Build history of the part. All positions in model axes, mm. A direction names the side the tool comes from. Give positions to 0.01 mm unless a question says otherwise; leave off trailing zeros. Order: outer loops, then holes, each group sorted by start corner. A loop starts at its lowest first (then second) coordinate and runs counter-clockwise, first axis right, second up. Notation, with made-up numbers: M -14.75,-11 L 26.25,-11 A9 ccw 26.25,-6 Z; hole C -38,40.5 d1. An arc over 180 degrees is marked long. Answer as CSV lines item,"result".
from build123d import *

# Parameters (mm, degrees)
RESSALTO_EXTRUS_O3_DEPTH = 5
ESBO_O4_R                = 1.5
CORTE_EXTRUS_O3_DEPTH    = 10
CORTE_EXTRUS_O4_DEPTH    = 10


with BuildPart() as part:
    # Esboço1 → Ressalto-extrusão3 (new body)
    with BuildSketch(Plane.XY):
        with BuildLine():
            Line((-31.851570772, -17.801096987), (-27.063885949, -17.801096987))
            Line((-27.063885949, -17.801096987), (10.936114051, -17.801096987))
            Line((10.936114051, -17.801096987), (15.723798874, -17.801096987))
            ThreePointArc((15.723798874, -17.801096987), (21.039894205, -19.331201448), (24.729153299, -23.4532709))
            ThreePointArc((24.729153299, -23.4532709), (27.934250919, -27.635644423), (32.536114051, -30.202306605))
            ThreePointArc((32.536114051, -30.202306605), (35.210937986, -29.759166326), (36.436114051, -27.340489001))
            Line((36.436114051, -27.340489001), (36.436114051, -17.801096987))
            Line((36.436114051, -17.801096987), (36.436114051, 0.198903013))
            add(Edge.make_bspline(
                [(36.436114051, 75.398903013), (24.729153299, 37.798903013), (36.436114051, 0.198903013)],
                knots=[0, 0, 0, 1, 1, 1], degree=2, weights=[1, 3, 1]))
            Line((36.436114051, 75.398903013), (36.436114051, 93.398903013))
            Line((36.436114051, 93.398903013), (36.436114051, 102.938295027))
            ThreePointArc((36.436114051, 102.938295027), (35.210937986, 105.356972352), (32.536114051, 105.800112631))
            ThreePointArc((32.536114051, 105.800112631), (27.934250919, 103.23345045), (24.729153299, 99.051076926))
            ThreePointArc((24.729153299, 99.051076926), (21.039894205, 94.929007474), (15.723798874, 93.398903013))
            Line((15.723798874, 93.398903013), (10.936114051, 93.398903013))
            Line((10.936114051, 93.398903013), (-27.063885949, 93.398903013))
            Line((-27.063885949, 93.398903013), (-31.851570772, 93.398903013))
            ThreePointArc((-31.851570772, 93.398903013), (-37.167666102, 94.929007474), (-40.856925197, 99.051076926))
            ThreePointArc((-40.856925197, 99.051076926), (-44.062022817, 103.23345045), (-48.663885949, 105.800112631))
            ThreePointArc((-48.663885949, 105.800112631), (-51.338709884, 105.356972352), (-52.563885949, 102.938295027))
            Line((-52.563885949, 102.938295027), (-52.563885949, 93.398903013))
            Line((-52.563885949, 93.398903013), (-52.563885949, 75.398903013))
            add(Edge.make_bspline(
                [(-52.563885949, 75.398903013), (-40.856925197, 37.798903013), (-52.563885949, 0.198903013)],
                knots=[0, 0, 0, 1, 1, 1], degree=2, weights=[1, 3, 1]))
            Line((-52.563885949, 0.198903013), (-52.563885949, -17.801096987))
            Line((-52.563885949, -17.801096987), (-52.563885949, -27.340489001))
            ThreePointArc((-52.563885949, -27.340489001), (-51.338709884, -29.759166326), (-48.663885949, -30.202306605))
            ThreePointArc((-48.663885949, -30.202306605), (-44.062022817, -27.635644423), (-40.856925197, -23.4532709))
            ThreePointArc((-40.856925197, -23.4532709), (-37.167666102, -19.331201448), (-31.851570772, -17.801096987))
        make_face()
    extrude(amount=RESSALTO_EXTRUS_O3_DEPTH)

    # Esboço4 → Corte-extrusão3 (cut)
    with BuildSketch(Plane(origin=(0, 0, 0), x_dir=(-1, 0, 0), z_dir=(0, 0, -1))):
        with Locations((-31.436114051, 99.800112631)):
            Circle(ESBO_O4_R)
        with Locations((47.563885949, 99.800112631)):
            Circle(ESBO_O4_R)
        with Locations((47.563885949, -24.202306605)):
            Circle(ESBO_O4_R)
        with Locations((-31.436114051, -24.202306605)):
            Circle(ESBO_O4_R)
        with BuildLine():
            Line((-12.436114051, 90.598903013), (-1.436114051, 90.598903013))
            ThreePointArc((-1.436114051, 90.598903013), (-0.021900489, 90.013116575), (0.563885949, 88.598903013))
            Line((0.563885949, 88.598903013), (0.563885949, 78.698903013))
            ThreePointArc((0.563885949, 78.698903013), (-0.021900489, 77.284689451), (-1.436114051, 76.698903013))
            Line((-1.436114051, 76.698903013), (-12.436114051, 76.698903013))
            ThreePointArc((-12.436114051, 76.698903013), (-13.850327613, 77.284689451), (-14.436114051, 78.698903013))
            Line((-14.436114051, 78.698903013), (-14.436114051, 88.598903013))
            ThreePointArc((-14.436114051, 88.598903013), (-13.850327613, 90.013116575), (-12.436114051, 90.598903013))
        make_face()
        with BuildLine():
            Line((17.563885949, 90.598903013), (28.563885949, 90.598903013))
            ThreePointArc((28.563885949, 90.598903013), (29.978099511, 90.013116575), (30.563885949, 88.598903013))
            Line((30.563885949, 88.598903013), (30.563885949, 78.698903013))
            ThreePointArc((30.563885949, 78.698903013), (29.978099511, 77.284689451), (28.563885949, 76.698903013))
            Line((28.563885949, 76.698903013), (17.563885949, 76.698903013))
            ThreePointArc((17.563885949, 76.698903013), (16.149672387, 77.284689451), (15.563885949, 78.698903013))
            Line((15.563885949, 78.698903013), (15.563885949, 88.598903013))
            ThreePointArc((15.563885949, 88.598903013), (16.149672387, 90.013116575), (17.563885949, 90.598903013))
        make_face()
        with BuildLine():
            Line((30.563885949, -13.001096987), (30.563885949, -3.101096987))
            ThreePointArc((30.563885949, -3.101096987), (29.978099511, -1.686883425), (28.563885949, -1.101096987))
            Line((28.563885949, -1.101096987), (17.563885949, -1.101096987))
            ThreePointArc((17.563885949, -1.101096987), (16.149672387, -1.686883425), (15.563885949, -3.101096987))
            Line((15.563885949, -3.101096987), (15.563885949, -13.001096987))
            ThreePointArc((15.563885949, -13.001096987), (16.149672387, -14.415310549), (17.563885949, -15.001096987))
            Line((17.563885949, -15.001096987), (28.563885949, -15.001096987))
            ThreePointArc((28.563885949, -15.001096987), (29.978099511, -14.415310549), (30.563885949, -13.001096987))
        make_face()
        with BuildLine():
            Line((0.563885949, -13.001096987), (0.563885949, -3.101096987))
            ThreePointArc((0.563885949, -3.101096987), (-0.021900489, -1.686883425), (-1.436114051, -1.101096987))
            Line((-1.436114051, -1.101096987), (-12.436114051, -1.101096987))
            ThreePointArc((-12.436114051, -1.101096987), (-13.850327613, -1.686883425), (-14.436114051, -3.101096987))
            Line((-14.436114051, -3.101096987), (-14.436114051, -13.001096987))
            ThreePointArc((-14.436114051, -13.001096987), (-13.850327613, -14.415310549), (-12.436114051, -15.001096987))
            Line((-12.436114051, -15.001096987), (-1.436114051, -15.001096987))
            ThreePointArc((-1.436114051, -15.001096987), (-0.021900489, -14.415310549), (0.563885949, -13.001096987))
        make_face()
    extrude(amount=-CORTE_EXTRUS_O3_DEPTH, mode=Mode.SUBTRACT)

    # Esboço5 → Corte-extrusão4 (cut)
    with BuildSketch(Plane.XY.offset(5)):
        with BuildLine():
            Line((2.436114051, 17.798903013), (12.436114051, 17.798903013))
            ThreePointArc((12.436114051, 17.798903013), (15.971647957, 19.263369107), (17.436114051, 22.798903013))
            Line((17.436114051, 22.798903013), (17.436114051, 52.798903013))
            ThreePointArc((17.436114051, 52.798903013), (15.971647957, 56.334436919), (12.436114051, 57.798903013))
            Line((12.436114051, 57.798903013), (2.436114051, 57.798903013))
            ThreePointArc((2.436114051, 57.798903013), (-1.099419855, 56.334436919), (-2.563885949, 52.798903013))
            Line((-2.563885949, 52.798903013), (-2.563885949, 22.798903013))
            ThreePointArc((-2.563885949, 22.798903013), (-1.099419855, 19.263369107), (2.436114051, 17.798903013))
        make_face()
    extrude(amount=-CORTE_EXTRUS_O4_DEPTH, mode=Mode.SUBTRACT)


solid = part.part
Item 1: Band-saw the part on B-B (y = -8). Give the cut face in (x, z).
Geometry says:
outline,"M -52.56,0 L -30.56,0 L -30.56,5 L -52.56,5 Z; M -15.56,0 L -0.56,0 L -0.56,5 L -15.56,5 Z; M 14.44,0 L 36.44,0 L 36.44,5 L 14.44,5 Z"
Item 2: 3-axis set-ups, long thin cutter, end or side, ignore diameter. For faces 4 (the cylindrical face through (27.88, -27.59, 2.46)), 5 (the flat face through (-8, 93.399, 2)), 6 (the flat face through (36.436, 89, 2)), 7 (the flat face through (-15.564, -8, 2)): which of +Z, -Z, +X, -X, +Y, -Y reach the whole face in a straight line?
Geometry says:
face 4,"+Z, -Z, -Y"
face 5,"+Z, -Z, +Y"
face 6,"+Z, -Z, +X, +Y, -Y"
face 7,"+Z, -Z"
Item 3: Band-saw the part on C-C (x = -27). Give the cut face in (y, z), and give its area (3 significant figures).
Geometry says:
outline,"M -17.8,0 L -15,0 L -15,5 L -17.8,5 Z; M -1.1,0 L 76.7,0 L 76.7,5 L -1.1,5 Z; M 90.6,0 L 93.4,0 L 93.4,5 L 90.6,5 Z"
area,"417 mm2"
Item 4: Probe line 1 along Y through (x, z) = (-21.5, 4.7); line 2 along Y through (x, z) = (6, 4.45); line 3 along X through (y, z) = (-8, 2). List the from-to ranges inside material, lowest first. Write a range as from..to.
Geometry says:
line 1,"y = -17.8..-15, -1.1..76.7, 90.6..93.4"
line 2,"y = -17.8..-15, -1.1..17.8, 57.8..76.7, 90.6..93.4"
line 3,"x = -52.56..-30.56, -15.56..-0.56, 14.44..36.44"
Item 5: Band-saw the part on D-D (z = 3.8). State how many separate pieces and enclosed holes the cut face has, and give its area (3 significant figures).
Geometry says:
separate pieces,"1"
enclosed holes,"9"
area,"8,040 mm2"
Item 6: Band-saw the part on A-A (x = 7). Give the cut face in (y, z).
Geometry says:
outline,"M -17.8,0 L -15,0 L -15,5 L -17.8,5 Z; M -1.1,0 L 17.8,0 L 17.8,5 L -1.1,5 Z; M 57.8,0 L 76.7,0 L 76.7,5 L 57.8,5 Z; M 90.6,0 L 93.4,0 L 93.4,5 L 90.6,5 Z"
Item 7: Drop flat-ended pins along their axis: pin 1 (1 mm diameter, centred on x = -24.5, z = 1.5, fed in from +Y); pin 2 (1.8 mm diameter, centred on x = -47.56, y = -24.2, fed in from +Z); pin 3 (1 mm diameter, centred on x = -34.5, z = 2, fed in from -Y); pin 4 (1 mm diameter, centred on x = 17.5, z = 3.5, fed in from -Y). Give the stop position or say it passes through.
Geometry says:
pin 1,"stops at y = 93.4"
pin 2,"passes through"
pin 3,"stops at y = -18.31"
pin 4,"stops at y = -18.06"
Item 8: Pull direction Y, two halves, no side cores. Call faces 1 (the flat face through (-23, 76.699, 2)), 2 (the flat face through (-9, 39, 5)), 3 (the cylindrical face through (-51.37, -29.736, 2.465)): released by +Y, released by -Y, zero draft, split by the parting line, or undercut.
Geometry says:
face 1,"undercut"
face 2,"zero draft"
face 3,"released by -Y"
